```python
from build123d import *

# Parameters (mm, degrees)
F0_R        = 1.25
F0_R_2      = 3
F1_DEPTH    = 3
F2_SIZE2    = 6.99999
F2_SIZE     = 2.99999
F2_2_SIZE2  = 6.99999
F2_2_SIZE   = 2.99999
F3_SIZE2    = 2.99999
F3_SIZE     = 3.99999
F4_T1_DEPTH = 178.8917354422
F4_T3_DEPTH = 181.0057878677
F5_T1_DEPTH = 74.4931306538
F6_T1_DEPTH = 53.4058582454
F6_T3_DEPTH = 54.4906885897
F6_T5_DEPTH = 53.4058582454
F6_T7_DEPTH = 54.4906885841
F7_R        = 2.75
F7_R_2      = 1.25
F8_DEPTH    = 1.9


# Not quite as in the source:
# - a fillet or chamfer that OpenCascade refuses, or shapes differently, is made with other operations: its cross-section is extruded or revolved along the edge and cut away or added
# - a fillet or chamfer is up to 0.001 mm smaller than in the source, because OpenCascade refuses the exact size


with BuildPart() as f1:
    # F0 (on Top) → F1 (new body)
    with BuildSketch(Plane.XY):
        Polygon((-44.1484891925, -17.5328822659), (-29.4527173684, -20.9256685242), (27.0472826316, -20.9256685242), (73.6322826316, -10.1706738406), (73.6322826316, 38.4598458413), (25.9902564184, 49.4588742547), (-28.3956911556, 49.4588742546), (-76.037717368, 38.4598458414), (-76.0377173684, -10.1706738406), align=None)
        with Locations((-68.7027173684, -8.6404804453)):
            Circle(F0_R, mode=Mode.SUBTRACT)
        with Locations((-23.7027173684, -8.6404804453)):
            Circle(F0_R, mode=Mode.SUBTRACT)
        with BuildLine():
            ThreePointArc((-27.0502267204, -2.2085264366), (-71.2027173684, 13.8595195547), (-27.0502267204, 29.927565546))
            Line((-27.0502267204, 29.927565546), (-27.0502267204, 28.3226486068))
            ThreePointArc((-27.0502267204, 28.3226486068), (-22.2027173684, 13.8595195547), (-27.0502267204, -0.6036094974))
            Line((-27.0502267204, -0.6036094974), (-27.0502267204, -2.2085264366))
        make_face(mode=Mode.SUBTRACT)
        with Locations((-11.7027286338, 1.5743587088)):
            Circle(F0_R_2, mode=Mode.SUBTRACT)
        with Locations((21.2972826316, -8.6404804453)):
            Circle(F0_R, mode=Mode.SUBTRACT)
        with Locations((66.2972826316, -8.6404804453)):
            Circle(F0_R, mode=Mode.SUBTRACT)
        with Locations((9.2972956984, 1.5743587088)):
            Circle(F0_R_2, mode=Mode.SUBTRACT)
        with BuildLine():
            ThreePointArc((24.6447919836, 29.927565546), (68.7972826316, 13.8595195547), (24.6447919836, -2.2085264366))
            Line((24.6447919836, -2.2085264366), (24.6447919836, -0.6036094974))
            ThreePointArc((24.6447919836, -0.6036094974), (19.7972826316, 13.8595195547), (24.6447919836, 28.3226486068))
            Line((24.6447919836, 28.3226486068), (24.6447919836, 29.927565546))
        make_face(mode=Mode.SUBTRACT)
        with BuildLine():
            Line((4.8972822306, 35.2537547127), (4.8972822306, 17.9537547127))
            ThreePointArc((4.8972822306, 17.9537547127), (4.1650491836, 16.1859877597), (2.3972822306, 15.4537547127))
            Line((2.3972822306, 15.4537547127), (-4.8027177694, 15.4537547127))
            ThreePointArc((-4.8027177694, 15.4537547127), (-6.5704847223, 16.1859877597), (-7.3027177694, 17.9537547127))
            Line((-7.3027177694, 17.9537547127), (-7.3027177694, 35.2537547127))
            ThreePointArc((-7.3027177694, 35.2537547127), (-6.5704847223, 37.0215216656), (-4.8027177694, 37.7537547127))
            Line((-4.8027177694, 37.7537547127), (2.3972822306, 37.7537547127))
            ThreePointArc((2.3972822306, 37.7537547127), (4.1650491836, 37.0215216656), (4.8972822306, 35.2537547127))
        make_face(mode=Mode.SUBTRACT)
        with Locations((-68.7027173684, 36.3595195547)):
            Circle(F0_R, mode=Mode.SUBTRACT)
        with Locations((-23.7027173684, 36.3595195547)):
            Circle(F0_R, mode=Mode.SUBTRACT)
        Polygon((-7.7027173684, 44.858563391), (5.2972826316, 44.858563391), (4.4972826316, 44.058563391), (-6.9027173684, 44.058563391), align=None, mode=Mode.SUBTRACT)
        Polygon((-9.2027173684, 46.658563391), (6.7972826316, 46.658563391), (5.9972826316, 45.858563391), (-8.4027173684, 45.858563391), align=None, mode=Mode.SUBTRACT)
        Polygon((-10.7027173684, 48.458563391), (8.2972826316, 48.458563391), (7.4972826316, 47.658563391), (-9.9027173684, 47.658563391), align=None, mode=Mode.SUBTRACT)
        with Locations((21.2972826316, 36.3595195547)):
            Circle(F0_R, mode=Mode.SUBTRACT)
        with Locations((66.2972826316, 36.3595195547)):
            Circle(F0_R, mode=Mode.SUBTRACT)
    extrude(amount=F1_DEPTH)

    # F2 (size 3 and 7 in the source; OpenCascade refuses exactly that, so slightly less here)
    f2_edges = [f1.edges().sort_by_distance(p)[0] for p in [
        (6.297296, 1.574359, 3),
    ]]
    f2_side = f1.faces().sort_by_distance((6.297296, 1.574359, 1.5))[0]
    chamfer(f2_edges, length=F2_SIZE, length2=F2_SIZE2, reference=f2_side)

    # F2#2 (size 3 and 7 in the source; OpenCascade refuses exactly that, so slightly less here)
    f2_2_edges = [f1.edges().sort_by_distance(p)[0] for p in [
        (-14.702729, 1.574359, 3),
    ]]
    f2_2_side = f1.faces().sort_by_distance((-14.702729, 1.574359, 1.5))[0]
    chamfer(f2_2_edges, length=F2_2_SIZE, length2=F2_2_SIZE2, reference=f2_2_side)

    # F3 (size 4 and 3 in the source; OpenCascade refuses exactly that, so slightly less here)
    f3_edges = [f1.edges().sort_by_distance(p)[0] for p in [
        (-1.202718, 37.753755, 3),
        (-7.302718, 26.603755, 3),
        (-1.202718, 15.453755, 3),
        (-6.570485, 16.185988, 3),
        (4.165049, 16.185988, 3),
        (4.897282, 26.603755, 3),
        (4.165049, 37.021522, 3),
        (-6.570485, 37.021522, 3),
    ]]
    f3_side = f1.faces().sort_by_distance((-1.202717, 15.209837, 3))[0]
    chamfer(f3_edges, length=F3_SIZE, length2=F3_SIZE2, reference=f3_side)

    # F4: chamfer of 3 x 8 on 2 edges, made by hand

    # F4_s2 → F4_t1 (cut)
    with BuildSketch(Plane.YZ.offset(-90.6485850894)):
        Polygon((41.4588742546, 3), (49.4588742546, 0), (49.4588742546, 3), align=None)
    extrude(amount=F4_T1_DEPTH, mode=Mode.SUBTRACT)

    # F4_s4 → F4_t3 (cut)
    with BuildSketch(Plane.YZ.offset(-91.7056113022)):
        Polygon((-12.9256685242, 3), (-20.9256685242, 0), (-20.9256685242, 3), align=None)
    extrude(amount=F4_T3_DEPTH, mode=Mode.SUBTRACT)

    # F5: chamfer of 5 x 3 on 2 edges, made by hand

    # F5_s2 → F5_t1 (cut)
    with BuildSketch(Plane.XZ.offset(-51.3911513272)):
        Polygon((-71.0377173684, 3), (-76.0377173684, 0), (-76.0377173684, 3), align=None)
        Polygon((68.6322826316, 3), (73.6322826316, 0), (73.6322826316, 3), align=None)
    extrude(amount=F5_T1_DEPTH, mode=Mode.SUBTRACT)

    # F6: chamfer of 3 on 4 edges, made by hand

    # F6_s2 → F6_t1 (cut)
    with BuildSketch(Plane(origin=(-20.4409607394, 4.7191676308, 0), x_dir=(0, 0, 1), z_dir=(-0.9743700648, 0.2249510543, 0))):
        Polygon((3, -24.0147648209), (0, -27.0147648209), (3, -27.0147648209), align=None)
    extrude(amount=F6_T1_DEPTH, mode=Mode.SUBTRACT)

    # F6_s4 → F6_t3 (cut)
    with BuildSketch(Plane(origin=(-13.1833561407, -3.0436175852, 0), x_dir=(0, 0, 1), z_dir=(-0.9743700648, -0.2249510543, 0))):
        Polygon((3, 51.5788871759), (0, 54.5788871759), (3, 54.5788871759), align=None)
    extrude(amount=F6_T3_DEPTH, mode=Mode.SUBTRACT)

    # F6_s6 → F6_t5 (cut)
    with BuildSketch(Plane(origin=(18.1572481609, 4.1919310387, 0), x_dir=(0, 0, 1), z_dir=(0.9743700648, 0.2249510543, 0))):
        Polygon((3, 23.4736597407), (0, 26.4736597407), (3, 26.4736597407), align=None)
    extrude(amount=F6_T5_DEPTH, mode=Mode.SUBTRACT)

    # F6_s8 → F6_t7 (cut)
    with BuildSketch(Plane(origin=(63.9937393355, -14.7741188415, 0), x_dir=(0, 0, 1), z_dir=(-0.9743700648, 0.2249510543, 0))):
        Polygon((3, 51.0377820952), (0, 54.0377820952), (3, 54.0377820952), align=None)
    extrude(amount=F6_T7_DEPTH, mode=Mode.SUBTRACT)

    # F7 (on face) → F8 (cut)
    with BuildSketch(Plane.XY.offset(3)):
        with Locations((-68.7027173684, 36.3595195547)):
            Circle(F7_R)
        with Locations((-68.7027173684, 36.3595195547)):
            Circle(F7_R_2, mode=Mode.SUBTRACT)
        with Locations((-23.7027173684, 36.3595195547)):
            Circle(F7_R)
        with Locations((-23.7027173684, 36.3595195547)):
            Circle(F7_R_2, mode=Mode.SUBTRACT)
        with Locations((21.2972826316, 36.3595195547)):
            Circle(F7_R)
        with Locations((21.2972826316, 36.3595195547)):
            Circle(F7_R_2, mode=Mode.SUBTRACT)
        with Locations((66.2972826316, 36.3595195547)):
            Circle(F7_R)
        with Locations((66.2972826316, 36.3595195547)):
            Circle(F7_R_2, mode=Mode.SUBTRACT)
        with Locations((66.2972826316, -8.6404804453)):
            Circle(F7_R)
        with Locations((66.2972826316, -8.6404804453)):
            Circle(F7_R_2, mode=Mode.SUBTRACT)
        with Locations((21.2972826316, -8.6404804453)):
            Circle(F7_R)
        with Locations((21.2972826316, -8.6404804453)):
            Circle(F7_R_2, mode=Mode.SUBTRACT)
        with Locations((-23.7027173684, -8.6404804453)):
            Circle(F7_R)
        with Locations((-23.7027173684, -8.6404804453)):
            Circle(F7_R_2, mode=Mode.SUBTRACT)
        with Locations((-68.7027173684, -8.6404804453)):
            Circle(F7_R)
        with Locations((-68.7027173684, -8.6404804453)):
            Circle(F7_R_2, mode=Mode.SUBTRACT)
    extrude(amount=-F8_DEPTH, mode=Mode.SUBTRACT)


solid = f1.part
```
Geometry check sheet. Reference: the model listing, model coordinates, mm. A direction names the side the tool comes from. Coordinates: 2 decimals unless noted, no trailing zeros. Loops run counter-clockwise (first coordinate to the right, second up) from the corner with the lowest first, then second, coordinate; pieces in that order, holes last. Notation, with made-up numbers: (-5.75, -13) -> (34.25, -13) arc R20 cw to (34.25, 11) -> close; hole circle Ø7 at (2.25, 13). An arc over 180 degrees is marked (long way). Put each result on its own line as item: value.
1) Cross-section at D-D on y = -16. Record the boundary of the cut face in (x, z).
Result set:
outline: (-50.79, 0) -> (48.38, 0) -> (40.17, 1.85) -> (-42.58, 1.85) -> close
2) Tool access check on faces 4 (the flat face through (-2, 10, 3)), 5 (the conical face through (-7.62, 15.07, 1.15)), 6 (the cylindrical face through (19.8, 13.6, 1.5)). Record the directions out of +Z, -Z, +X, -X, +Y, -Y that give a thin tool (end or side, any length) a straight path to the whole face; none if there is none.
Result set:
face 4: +Z, +X, -X, +Y, -Y
face 5: +Z
face 6: +Z, -Z
3) Cross-section at B-B on x = 50.5. Record the boundary of the cut face in (y, z), plus the area to 3 significant figures.
Result set:
outline: (-15.51, 0) -> (-10.23, 0) -> (-10.23, 3) -> (-12.43, 3) -> close; (37.94, 0) -> (43.8, 0) -> (40.72, 3) -> (37.94, 3) -> close
area: 24.2 mm^2
4) Thickness scan on line 1 (X direction, y = 28, z = 1.2); line 2 (X direction, y = 21, z = 0.4); line 3 (X direction, y = -4, z = 0.8). Record the ranges inside material, lowest first.
Result set:
line 1: x = -74.04 to -66.82, -26.81 to -8.9, 6.5 to 24.41, 64.41 to 71.63
line 2: x = -75.37 to -70.16, -23.29 to -7.84, 5.43 to 20.88, 67.76 to 72.97
line 3: x = -74.7 to -63.7, -28.71 to 26.3, 61.29 to 72.3
5) Release check for a two-part mould opening along Y. For faces 1 (the flat face through (67, 35, 1.1)), 2 (the flat face through (71.1, 14.48, 1.52)), 3 (the flat face through (-56.91, 41.657, 1.188)) record: released by +Y, released by -Y, zero draft, split by the parting line, or undercut.
Result set:
face 1: undercut
face 2: zero draft
face 3: released by +Y
6) Gauge pin test, flat ends, axial feed: pin 1 Ø0.6 at (x, z) = (-2, 1.5) entering from +Y; pin 2 Ø3 at (x, y) = (21, -9) entering from +Z; pin 3 Ø0.8 at (y, z) = (-1.5, 1.5) entering from +X. Record the tip position at first contact, or that the pin passes through.
Result set:
pin 1: stops at y = 45.86
pin 2: stops at z = 1.1
pin 3: stops at x = 71.8
7) Cross-section at A-A on y = 24. Count the separate pieces of the cut face and the enclosed holes in it, plus the area to 3 significant figures.
Result set:
separate pieces: 4
enclosed holes: 0
area: 118 mm^2
